from build123d import *

# Parameters (mm, degrees)
BOSS_EXTRU_2_DEPTH      = 10.4
ESQUISSE2_R             = 2.5
ENL_V_MAT_EXTRU_1_DEPTH = 2.5
ENL_V_MAT_EXTRU_2_DEPTH = 1.9
ENL_V_MAT_EXTRU_3_DEPTH = 3
ESQUISSE6_R             = 2.625
ENL_V_MAT_EXTRU_4_DEPTH = 77.245393303
ESQUISSE8_W             = 4.091090074
ESQUISSE8_H             = 23.887427299
ENL_V_MAT_EXTRU_5_DEPTH = 79
ENL_V_MAT_EXTRU_6_REACH = 78.075
ESQUISSE9_R             = 2.5
CONG_2_R                = 1
CONG_3_R                = 1


with BuildPart() as part:
    # Esquisse1 → Boss.-Extru.2 (new body)
    with BuildSketch(Plane.XY):
        with BuildLine():
            Line((44.737484162, 10), (65, 10))
            ThreePointArc((65, 10), (75, 0), (65, -10))
            Line((65, -10), (44.737484162, -10))
            ThreePointArc((44.737484162, -10), (42.506197266, -9.916907574), (40.287270574, -9.668090586))
            Line((40.287270574, -9.668090586), (10.054978641, -5.133246796))
            ThreePointArc((10.054978641, -5.133246796), (8.226779369, -4.12410675), (7.5, -2.166437738))
            Line((7.5, -2.166437738), (7.5, 2.166437738))
            ThreePointArc((7.5, 2.166437738), (8.226779369, 4.12410675), (10.054978641, 5.133246796))
            Line((10.054978641, 5.133246796), (40.287270574, 9.668090586))
            ThreePointArc((40.287270574, 9.668090586), (42.506197266, 9.916907574), (44.737484162, 10))
        make_face()
    extrude(amount=BOSS_EXTRU_2_DEPTH)

    # Esquisse2 → Enlèv. mat.-Extru.1 (cut)
    with BuildSketch(Plane.XY.offset(10.4)):
        with Locations((65, 0)):
            Circle(ESQUISSE2_R)
    extrude(amount=-ENL_V_MAT_EXTRU_1_DEPTH, mode=Mode.SUBTRACT)

    # Esquisse3 → Enlèv. mat.-Extru.2 (cut)
    with BuildSketch(Plane.XY.offset(5.9)):
        with BuildLine():
            Line((87.5, 3.75), (87.5, -3.75))
            Line((87.5, -3.75), (65, -3.75))
            Line((65, -3.75), (65, -3.5))
            ThreePointArc((65, -3.5), (64.812229587, -3.494959552), (64.625, -3.479852727))
            Line((64.625, -3.479852727), (50.785714286, -1.988487272))
            ThreePointArc((50.785714286, -1.988487272), (49, 0), (50.785714286, 1.988487272))
            Line((50.785714286, 1.988487272), (64.625, 3.479852727))
            ThreePointArc((64.625, 3.479852727), (64.812229587, 3.494959552), (65, 3.5))
            Line((65, 3.5), (65, 3.75))
            Line((65, 3.75), (87.5, 3.75))
        make_face()
    extrude(amount=-ENL_V_MAT_EXTRU_2_DEPTH, mode=Mode.SUBTRACT)

    # Esquisse4 → Enlèv. mat.-Extru.3 (cut)
    with BuildSketch(Plane.XY.offset(4)):
        with BuildLine():
            Line((65, 3.5), (65, 3.75))
            Line((65, 3.75), (88.077593775, 3.75))
            Line((88.077593775, 3.75), (88.077593775, -3.75))
            Line((88.077593775, -3.75), (65, -3.75))
            Line((65, -3.75), (65, -3.5))
            ThreePointArc((65, -3.5), (61.5, 0), (65, 3.5))
        make_face()
    extrude(amount=-ENL_V_MAT_EXTRU_3_DEPTH, mode=Mode.SUBTRACT)

    # Esquisse6 → Enlèv. mat.-Extru.4 (cut, through all)
    with BuildSketch(Plane.XY.offset(1)):
        with Locations((65, 0)):
            Circle(ESQUISSE6_R)
    extrude(amount=-ENL_V_MAT_EXTRU_4_DEPTH, mode=Mode.SUBTRACT)

    # Esquisse8 → Enlèv. mat.-Extru.5 (cut)
    with BuildSketch(Plane(origin=(0, 0, 0), x_dir=(0, 0, -1), z_dir=(1, 0, 0))):
        with Locations((-9.945545037, 0.586827687)):
            Rectangle(ESQUISSE8_W, ESQUISSE8_H)
    extrude(amount=ENL_V_MAT_EXTRU_5_DEPTH, mode=Mode.SUBTRACT)

    # Esquisse9 → Enlèv. mat.-Extru.6 (cut, up to next)
    with BuildSketch(Plane.XY.offset(7.9), mode=Mode.PRIVATE) as enl_v_mat_extru_6_sk1:
        with Locations((65, 0)):
            Circle(ESQUISSE9_R)
    enl_v_mat_extru_6_tool1 = extrude(enl_v_mat_extru_6_sk1.sketch, amount=-ENL_V_MAT_EXTRU_6_REACH, mode=Mode.PRIVATE) & part.part
    add(enl_v_mat_extru_6_tool1.solids().sort_by_distance((65, 0, 7.9))[0], mode=Mode.SUBTRACT)

    # Congé2
    cong_2_edges = [part.edges().sort_by_distance(p)[0] for p in [
        (8.226779369, -4.12410675, 7.9),
        (25.171124608, -7.400668691, 7.9),
        (42.506197266, -9.916907574, 7.9),
        (54.868742081, -10, 7.9),
        (75, 0, 7.9),
        (54.868742081, 10, 7.9),
        (42.506197266, 9.916907574, 7.9),
        (25.171124608, 7.400668691, 7.9),
        (8.226779369, 4.12410675, 7.9),
        (7.5, 0, 7.9),
        (62.5, 0, 7.9),
    ]]
    fillet(cong_2_edges, radius=CONG_2_R)

    # Congé3
    cong_3_edges = [part.edges().sort_by_distance(p)[0] for p in [
        (7.5, 0, 0),
        (8.226779369, 4.12410675, 0),
        (25.171124608, 7.400668691, 0),
        (42.506197266, 9.916907574, 0),
        (54.868742081, 10, 0),
        (75, 0, 0),
        (54.868742081, -10, 0),
        (42.506197266, -9.916907574, 0),
        (25.171124608, -7.400668691, 0),
        (8.226779369, -4.12410675, 0),
        (62.375, 0, 0),
    ]]
    fillet(cong_3_edges, radius=CONG_3_R - 0.0001)  # a hair under: the kernel refuses the full size


solid = part.part
Could you check a few things on this model? Use its own coordinates, in mm. A direction names the side the tool comes from. Round coordinates to 2 decimals unless told otherwise and drop trailing zeros. Write each loop counter-clockwise with the first axis right and the second up, starting at its lowest first coordinate (ties: lowest second). Pieces come first, ordered by that corner, then holes. Notation, with made-up numbers: (33, 18.5) - (46, 18.5) arc R38 ccw to (46, 56.5) - close; hole circle Ø7 at (59.25, -13). An arc over 180 degrees is marked (long way). Put each result on its own line as item: value. Start each with the question number.
(1) Thinking about a two-plate mould opening in Z: for faces 1 (the flat face through (57.802, -2.745, 4.963)), 2 (the flat face through (55, 10, 4)), 3 (the flat face through (41, 0, 7.9)), which applies, released by +Z, released by -Z, zero draft, split by the parting line, or undercut?
(2) I want a section at A-A, the plane y = 0. Give the number of separate pieces and of enclosed holes in the cut face, plus the area to 3 significant figures.
(3) For faces 4 (the flat face through (24.96, 7.37, 3.91)), 5 (the flat face through (57.608, 2.724, 4.963)), which set-ups out of +Z, -Z, +X, -X, +Y, -Y let a thin tool reach every point of the face, with its end or its side?
(4) I want a section at B-B, the plane x = 51.5. Please give me the cut outline in (y, z), plus the area to 3 significant figures.
(5) I need wall thicknesses on probe 1 along Y at (x, z) = (65, 6.3); probe 2 along X at (y, z) = (-0.25, 6.5); probe 3 along X at (y, z) = (0, 1.05). Which ranges of each line are inside material? Lowest first, please.
(6) I want a section at C-C, the plane z = 3. Please give me the cut outline in (x, y).
(7) Will these pins go through, and if not, where does the flat tip stop? pin 1 (2.5 mm diameter, centred on x = 72, z = 2.5, fed in from +Y); pin 2 (2 mm diameter, centred on x = 40.5, z = 4, fed in from -Y); pin 3 (1 mm diameter, centred on y = 7, z = 2, fed in from +X).
Here are the results:
1. face 1: undercut
1. face 2: zero draft
1. face 3: released by +Z
2. separate pieces: 3
2. enclosed holes: 0
2. area: 426 mm^2
3. face 4: +Z, -Z, -X, +Y
3. face 5: +X
4. outline: (-10, 1) arc R1 ccw to (-9, 0) - (9, 0) arc R1 ccw to (10, 1) - (10, 6.9) arc R1 ccw to (9, 7.9) - (-9, 7.9) arc R1 ccw to (-10, 6.9) - close; hole (-2.07, 4) - (2.07, 4) - (2.07, 5.9) - (-2.07, 5.9) - close
4. area: 149 mm^2
5. probe 1: y = -10 to -2.5, 2.5 to 10
5. probe 2: x = 7.5 to 62.51, 67.49 to 75
5. probe 3: x = 7.5 to 61.5
6. outline: (7.5, -2.17) arc R3 ccw to (10.05, -5.13) - (40.29, -9.67) arc R30 ccw to (44.74, -10) - (65, -10) arc R10 ccw to (74.27, -3.75) - (65, -3.75) - (65, -3.5) arc R3.5 cw to (65, 3.5) - (65, 3.75) - (74.27, 3.75) arc R10 ccw to (65, 10) - (44.74, 10) arc R30 ccw to (40.29, 9.67) - (10.05, 5.13) arc R3 ccw to (7.5, 2.17) - close
7. pin 1: stops at y = 8.18
7. pin 2: stops at y = -9.82
7. pin 3: stops at x = 72.6
